```python
from build123d import *

# Parameters (mm, degrees)
SKETCH1_W           = 406.4
SKETCH1_H           = 50.8
SKETCH1_W_2         = 101.6
BOSS_EXTRUDE1_DEPTH = 2.54
SKETCH2_R           = 2.794
CUT_EXTRUDE1_DEPTH  = 2.54
FILLET1_R           = 12.7
FILLET2_R           = 12.7


with BuildPart() as part:
    # Sketch1 → Boss-Extrude1 (new body)
    with BuildSketch(Plane(origin=(0, 0, 0), x_dir=(1, 0, 0), z_dir=(0, 1, 0))):
        with Locations((203.2, 25.4)):
            Rectangle(SKETCH1_W, SKETCH1_H)
        with Locations((203.2, 76.2)):
            Rectangle(SKETCH1_W_2, SKETCH1_H)
    extrude(amount=BOSS_EXTRUDE1_DEPTH)

    # Sketch2 → Cut-Extrude1 (cut)
    with BuildSketch(Plane(origin=(0, 2.54, 0), x_dir=(1, 0, 0), z_dir=(0, 1, 0))):
        with Locations(Location((222.25, 76.2, 0), (0, 0, 270))):
            Circle(SKETCH2_R)
        with Locations(Location((184.15, 76.2, 0), (0, 0, 270))):
            Circle(SKETCH2_R)
    extrude(amount=-CUT_EXTRUDE1_DEPTH, mode=Mode.SUBTRACT)

    # Fillet1
    fillet1_edges = [part.edges().sort_by_distance(p)[0] for p in [
        (152.4, 1.27, -101.6),
        (254, 1.27, -101.6),
    ]]
    fillet(fillet1_edges, radius=FILLET1_R)

    # Fillet2
    fillet2_edges = [part.edges().sort_by_distance(p)[0] for p in [
        (152.4, 1.27, -50.8),
        (254, 1.27, -50.8),
    ]]
    fillet(fillet2_edges, radius=FILLET2_R)


solid = part.part
```
Check sheet for the modelled part. Datum: model origin and axes. Units: mm. Coordinates: 2 decimals unless noted, no trailing zeros. Write each loop counter-clockwise with the first axis right and the second up, starting at its lowest first coordinate (ties: lowest second). Pieces come first, ordered by that corner, then holes. Notation, with made-up numbers: M 15.5,-28 L 57.5,-28 A24 cw 57.5,-13 Z; hole C 80,-11 d5. An arc over 180 degrees is marked long. Write item = value, one per line. Start each with the question number.
1. Go/stop test with flat-tipped pins: pin 1 (1.5 mm diameter, centred on y = 2, z = -90, fed in from +X); pin 2 (0.8 mm diameter, centred on x = 60.5, y = 1, fed in from -Z); pin 3 (4.5 mm diameter, centred on x = 222.25, z = -76.2, fed in from -Y). Record where each tip stops, or that it passes through.
2. Sectioned sample at B-B (x = 70). Record the cut outline in (y, z), then the cut area to 3 significant figures.
3. Thickness scan on probe 1 along X at (y, z) = (1.25, -76.2); probe 2 along Z at (x, y) = (184.15, 0.85); probe 3 along X at (y, z) = (0.8, -77.5). Record the ranges inside material, lowest first.
4. Sectioned sample at A-A (y = 1.1). Record the cut outline in (x, z).
The answers:
q1.pin_1 = 254
q1.pin_2 = -50.8
q1.pin_3 = through
q2.outline = M 0,-50.8 L 2.54,-50.8 L 2.54,0 L 0,0 Z
q2.area = 129 mm²
q3.probe_1 = 152.4 to 181.36, 186.94 to 219.46, 225.04 to 254
q3.probe_2 = -101.6 to -78.99, -73.41 to 0
q3.probe_3 = 152.4 to 181.68, 186.62 to 219.78, 224.72 to 254
q4.outline = M 0,-50.8 L 139.7,-50.8 A12.7 cw 152.4,-63.5 L 152.4,-88.9 A12.7 ccw 165.1,-101.6 L 241.3,-101.6 A12.7 ccw 254,-88.9 L 254,-63.5 A12.7 cw 266.7,-50.8 L 406.4,-50.8 L 406.4,0 L 0,0 Z; hole C 184.15,-76.2 d5.59; hole C 222.25,-76.2 d5.59
